```python
from build123d import *

# Parameters (mm, degrees)
SKETCH2_R           = 8
SKETCH2_R_2         = 6
SKETCH2_W           = 5
SKETCH2_H           = 5
BOSS_EXTRUDE1_DEPTH = 3


with BuildPart() as part:
    # Sketch2 → Boss-Extrude1 (new body)
    with BuildSketch(Plane.XY):
        with BuildLine():
            Line((81.032103119, 50.181312), (81.032103119, 60.181312))
            Line((81.032103119, 60.181312), (78.032103119, 60.181312))
            Line((78.032103119, 60.181312), (78.032103119, 71.181312))
            ThreePointArc((78.032103119, 71.181312), (53.908058205, 79.251221529), (28.494548306, 78.134755037))
            ThreePointArc((28.494548306, 78.134755037), (13.721692274, 80.8793749), (-1.279201176, 80.017163065))
            ThreePointArc((-1.279201176, 80.017163065), (2.677054283, 70.700200378), (8.902417187, 62.718809041))
            ThreePointArc((8.902417187, 62.718809041), (5.05730693, 41.181312), (8.902417187, 19.643814959))
            ThreePointArc((8.902417187, 19.643814959), (2.677054283, 11.662423622), (-1.279201176, 2.345460935))
            ThreePointArc((-1.279201176, 2.345460935), (13.721692274, 1.4832491), (28.494548306, 4.227868963))
            ThreePointArc((28.494548306, 4.227868963), (53.908058205, 3.111402471), (78.032103119, 11.181312))
            Line((78.032103119, 11.181312), (78.032103119, 22.181312))
            Line((78.032103119, 22.181312), (81.032103119, 22.181312))
            Line((81.032103119, 22.181312), (81.032103119, 32.181312))
            Line((81.032103119, 32.181312), (78.032103119, 32.181312))
            Line((78.032103119, 32.181312), (78.032103119, 50.181312))
            Line((78.032103119, 50.181312), (81.032103119, 50.181312))
        make_face()
        with Locations((23.507028058, 53.931312)):
            Circle(SKETCH2_R, mode=Mode.SUBTRACT)
        with Locations((43.507028058, 41.181312)):
            Circle(SKETCH2_R_2, mode=Mode.SUBTRACT)
        with Locations((23.507028058, 28.431312)):
            Circle(SKETCH2_R, mode=Mode.SUBTRACT)
        with Locations((64.423022125, 41.181312)):
            Rectangle(SKETCH2_W, SKETCH2_H, mode=Mode.SUBTRACT)
        with Locations((64.423022125, 33.181312)):
            Rectangle(SKETCH2_W, SKETCH2_H, mode=Mode.SUBTRACT)
        Polygon((72.266288865, 48.59637551), (67.936161846, 46.09637551), (70.436161846, 41.766248491), (74.766288865, 44.266248491), align=None, mode=Mode.SUBTRACT)
        Polygon((67.936161846, 36.266248491), (72.266288865, 33.766248491), (74.766288865, 38.09637551), (70.436161846, 40.596375509), align=None, mode=Mode.SUBTRACT)
        with Locations((64.423022125, 49.181312)):
            Rectangle(SKETCH2_W, SKETCH2_H, mode=Mode.SUBTRACT)
        Polygon((56.579755385, 33.766248491), (60.909882404, 36.266248491), (58.409882404, 40.59637551), (54.079755385, 38.09637551), align=None, mode=Mode.SUBTRACT)
        Polygon((60.909882404, 46.09637551), (56.579755385, 48.596375509), (54.079755385, 44.266248491), (58.409882404, 41.766248491), align=None, mode=Mode.SUBTRACT)
    extrude(amount=BOSS_EXTRUDE1_DEPTH)


solid = part.part
```
Here's how the part is built. I have some questions about the finished solid (model axes, mm). A direction names the side the tool comes from. Round coordinates to 2 decimals unless told otherwise and drop trailing zeros. Order: outer loops, then holes, each group sorted by start corner. A loop starts at its lowest first (then second) coordinate and runs counter-clockwise, first axis right, second up. Notation, with made-up numbers: M 26,47 L 82,47 A20 ccw 82,83 Z; hole C 58,60 d6. An arc over 180 degrees is marked long. Answer as CSV lines item,"result".
Item 1: Please list where these lines run through material, in increasing order: L1, parallel to Y at x = 55, z = 2.55; L2, parallel to Y at x = 30.5, z = 2.35; L3, parallel to Y at x = 66.5, z = 0.1. Write a range as [from, to].
From the geometry:
L1,"[3.27, 36.5], [38.63, 43.73], [45.86, 79.09]"
L2,"[3.8, 24.55], [32.32, 50.05], [57.82, 78.57]"
L3,"[6.09, 30.68], [35.68, 38.68], [43.68, 46.68], [51.68, 76.27]"
Item 2: Imagine slicing it at C-C on x = 39. List the corners of the cut face in (y, z) for me.
From the geometry:
outline,"M 2.63,0 L 37.22,0 L 37.22,3 L 2.63,3 Z; M 45.14,0 L 79.73,0 L 79.73,3 L 45.14,3 Z"
Item 3: Imagine slicing it at A-A on y = 25.5. List the corners of the cut face in (x, z) for me.
From the geometry:
outline,"M 7.07,0 L 16.06,0 L 16.06,3 L 7.07,3 Z; M 30.95,0 L 81.03,0 L 81.03,3 L 30.95,3 Z"
Item 4: Imagine slicing it at D-D on z = 0.9. Give the number of separate pieces and of enclosed holes in the cut face, and give its area (3 significant figures).
From the geometry:
separate pieces,"1"
enclosed holes,"10"
area,"4,860 mm2"
Item 5: Which directions (+Z, -Z, +X, -X, +Y, -Y) give clear straight access to the entire face, cutting with the end or side of a thin tool? Please do faces 4 (the flat face through (80, 32.181, 1)), 5 (the cylindrical face through (13.932, 80.866, 1.479)), 6 (the flat face through (64, 51.681, 1)).
From the geometry:
face 4,"+Z, -Z, +X"
face 5,"+Z, -Z, +Y"
face 6,"+Z, -Z"
Item 6: For pin 1 (1.5 mm diameter, centred on y = 32, z = 1, fed in from -X); pin 2 (1 mm diameter, centred on x = 60.5, z = 2.5, fed in from +Y); pin 3 (1.5 mm diameter, centred on x = 80, z = 1, fed in from -Y), each with a flat end and sliding along its axis, tell me the tip position at first contact or that it passes through.
From the geometry:
pin 1,"x = 5.63"
pin 2,"y = 78.12"
pin 3,"y = 22.18"
Item 7: Imagine slicing it at B-B on x = 25. List the corners of the cut face in (y, z) for me.
From the geometry:
outline,"M 3.24,0 L 20.57,0 L 20.57,3 L 3.24,3 Z; M 36.29,0 L 46.07,0 L 46.07,3 L 36.29,3 Z; M 61.79,0 L 79.12,0 L 79.12,3 L 61.79,3 Z"
Item 8: We'd pull the mould along Y, two halves only. Please class faces 1 (the flat face through (81.032, 27, 1)), 2 (the flat face through (66.923, 33, 1)), 3 (the cylindrical face through (13.51, 1.47, 1.48)): +Y half, -Y half, draft (parallel to the pull), parting line (faces both ways), or undercut.
From the geometry:
face 1,"draft"
face 2,"undercut"
face 3,"-Y half"
